from build123d import *

# Parameters (mm, degrees)
SKETCH_1_R          = 4.5
SKETCH_1_R_2        = 2.05
EXTRUDE_1_DEPTH     = 6
SKETCH_2_R          = 4
CUT_EXTRUDE_1_DEPTH = 2
SKETCH_3_R          = 6.65
CUT_EXTRUDE_2_DEPTH = 3.9
SKETCH_4_R          = 7.65
CUT_EXTRUDE_3_DEPTH = 1.5
SKETCH_5_R          = 6
SKETCH_5_R_2        = 2.05
EXTRUDE_2_DEPTH     = 5.1


with BuildPart() as part:
    # 草图1 → 凸台-拉伸1 (new body)
    with BuildSketch(Plane(origin=(0, 0, 0), x_dir=(1, 0, 0), z_dir=(0, 1, 0))):
        with BuildLine():
            Line((-14.168368772, -10.096516067), (29.831631228, -10.096516067))
            ThreePointArc((29.831631228, -10.096516067), (35.831631228, -4.096516067), (29.831631228, 1.903483933))
            Line((29.831631228, 1.903483933), (20.297540319, 1.903483933))
            ThreePointArc((20.297540319, 1.903483933), (16.762006413, 3.367950028), (15.297540319, 6.903483933))
            Line((15.297540319, 6.903483933), (15.297540319, 13.790407079))
            ThreePointArc((15.297540319, 13.790407079), (3.297540319, 25.790407079), (-8.702459681, 13.790407079))
            Line((-8.702459681, 13.790407079), (-8.702459681, 6.903483933))
            ThreePointArc((-8.702459681, 6.903483933), (-10.166925775, 3.367950028), (-13.702459681, 1.903483933))
            Line((-13.702459681, 1.903483933), (-14.168368772, 1.903483933))
            ThreePointArc((-14.168368772, 1.903483933), (-20.168368772, -4.096516067), (-14.168368772, -10.096516067))
        make_face()
        with Locations(Location((3.297540319, 13.790407079, 0), (0, 0, 270))):
            Circle(SKETCH_1_R, mode=Mode.SUBTRACT)
        with Locations(Location((-14.168368772, -4.096516067, 0), (0, 0, 270))):
            Circle(SKETCH_1_R_2, mode=Mode.SUBTRACT)
        with Locations(Location((29.831631228, -4.096516067, 0), (0, 0, 270))):
            Circle(SKETCH_1_R_2, mode=Mode.SUBTRACT)
    extrude(amount=EXTRUDE_1_DEPTH)

    # 草图2 → 切除-拉伸1 (cut)
    with BuildSketch(Plane.XZ):
        with Locations(Location((-14.168368772, 4.096516067, 0), (0, 0, 270))):
            Circle(SKETCH_2_R)
        with Locations(Location((29.831631228, 4.096516067, 0), (0, 0, 270))):
            Circle(SKETCH_2_R)
    extrude(amount=-CUT_EXTRUDE_1_DEPTH, mode=Mode.SUBTRACT)

    # 草图3 → 切除-拉伸2 (cut)
    with BuildSketch(Plane(origin=(0, 6, 0), x_dir=(1, 0, 0), z_dir=(0, 1, 0))):
        with Locations(Location((3.297540319, 13.790407079, 0), (0, 0, 270))):
            Circle(SKETCH_3_R)
    extrude(amount=-CUT_EXTRUDE_2_DEPTH, mode=Mode.SUBTRACT)

    # 草图4 → 切除-拉伸3 (cut)
    with BuildSketch(Plane(origin=(0, 6, 0), x_dir=(1, 0, 0), z_dir=(0, 1, 0))):
        with Locations(Location((3.297540319, 13.790407079, 0), (0, 0, 270))):
            Circle(SKETCH_4_R)
    extrude(amount=-CUT_EXTRUDE_3_DEPTH, mode=Mode.SUBTRACT)

    # 草图5 → 凸台-拉伸2 (add)
    with BuildSketch(Plane(origin=(0, 6, 0), x_dir=(1, 0, 0), z_dir=(0, 1, 0))):
        with Locations(Location((29.831631228, -4.096516067, 0), (0, 0, 270))):
            Circle(SKETCH_5_R)
        with Locations(Location((29.831631228, -4.096516067, 0), (0, 0, 90))):
            Circle(SKETCH_5_R_2, mode=Mode.SUBTRACT)
    extrude(amount=EXTRUDE_2_DEPTH)


solid = part.part
Read the model definition and answer for the solid it produces. Units are mm, in the model's axes. A direction names the side the tool comes from. Give positions to 0.01 mm unless a question says otherwise; leave off trailing zeros. Write each loop counter-clockwise with the first axis right and the second up, starting at its lowest first coordinate (ties: lowest second). Pieces come first, ordered by that corner, then holes. Notation, with made-up numbers: (-2, 27.25) - (26, 27.25) arc R21 ccw to (26, 38.25) - close; hole circle Ø10 at (41, 72). An arc over 180 degrees is marked (long way). Return JSON: item names as keys, results as strings.
Q1. A cutting plane is placed at D-D, the plane z = 4. Determine the outline of the cut face in (x, y), and give its area (3 significant figures).
Reply:
{"outline": "(-20.17, 0) - (-18.17, 0) - (-18.17, 2) - (-16.22, 2) - (-16.22, 6) - (-20.17, 6) - close; (-12.12, 2) - (-10.17, 2) - (-10.17, 0) - (25.83, 0) - (25.83, 2) - (27.78, 2) - (27.78, 11.1) - (23.83, 11.1) - (23.83, 6) - (-12.12, 6) - close; (31.88, 2) - (33.83, 2) - (33.83, 0) - (35.83, 0) - (35.83, 11.1) - (31.88, 11.1) - close", "area": "312 mm²"}
Q2. A cutting plane is placed at B-B, the plane z = -10.5. Determine the outline of the cut face in (x, y).
Reply:
{"outline": "(-8.7, 0) - (0.23, 0) - (0.23, 2.1) - (-2.48, 2.1) - (-2.48, 4.5) - (-3.61, 4.5) - (-3.61, 6) - (-8.7, 6) - close; (6.37, 0) - (15.3, 0) - (15.3, 6) - (10.2, 6) - (10.2, 4.5) - (9.08, 4.5) - (9.08, 2.1) - (6.37, 2.1) - close"}
Q3. A cutting plane is placed at C-C, the plane x = 30.5. Determine the outline of the cut face in (y, z).
Reply:
{"outline": "(0, -1.87) - (11.1, -1.87) - (11.1, 2.16) - (2, 2.16) - (2, 0.15) - (0, 0.15) - close; (0, 8.04) - (2, 8.04) - (2, 6.03) - (11.1, 6.03) - (11.1, 10.06) - (0, 10.06) - close"}
Q4. A cutting plane is placed at A-A, the plane y = 3. Determine the outline of the cut face in (x, z), and give its area (3 significant figures).
Reply:
{"outline": "(-14.17, -1.9) - (-13.7, -1.9) arc R5 cw to (-8.7, -6.9) - (-8.7, -13.79) arc R12 ccw to (15.3, -13.79) - (15.3, -6.9) arc R5 cw to (20.3, -1.9) - (29.83, -1.9) arc R6 ccw to (29.83, 10.1) - (-14.17, 10.1) arc R6 ccw to start; hole circle Ø4.1 at (-14.17, 4.1); hole circle Ø13.3 at (3.3, -13.79); hole circle Ø4.1 at (29.83, 4.1)", "area": "998 mm²"}
Q5. For a pull along Z with two mould halves and no side action, classify faces 6 (the face through (0.368, 5.26, -6.724)), 7 (the face through (-20.167, 2.958, 3.965)), 8 (the face through (-10.128, 2.958, -3.407)), 9 (the face through (0.56, 1.04, -17.36)) as released by +Z, released by -Z, zero draft, split by the parting line, or undercut.
Reply:
{"face 6": "undercut", "face 7": "split by the parting line", "face 8": "released by -Z", "face 9": "undercut"}
Q6. Given P1, Ø4, axis at x = 20.5, y = 2, coming from the -Z side; P2, Ø4, axis at x = 28.5, z = 4, coming from the -Y side; P3, Ø11, axis at x = -6.5, z = 0, coming from the +Y side, each flat-ended and moving along its own axis, determine where each tip first touches the part or whether it passes through.
Reply:
{"P1": "z = -2.24", "P2": "y = 2", "P3": "y = 6"}
Q7. For faces 1 (the face through (-16.17, 3.97, 3.65)), 2 (the face through (-17.717, 0.986, 2.251)), 3 (the face through (25, 3, -1.903)), 4 (the face through (-8.702, 3, -10)), 5 (the face through (10, 4.5, -16)), determine the directions among +Z, -Z, +X, -X, +Y, -Y from which every point of the face is accessible in a straight line to the end or side of a thin tool.
Reply:
{"face 1": "+Y, -Y", "face 2": "-Y", "face 3": "-Z, +X, +Y, -Y", "face 4": "-Z, -X, +Y, -Y", "face 5": "+Y"}
Q8. Consider line 1 along Z through (x, y) = (-14, 2.5); line 2 along X through (y, z) = (1.5, -8); line 3 along Y through (x, z) = (-14, -0.5). Determine where each line is inside the solid, lowest interval first. Write a range as [from, to].
Reply:
{"line 1": "[-1.9, 2.05], [6.14, 10.1]", "line 2": "[-8.7, 15.3]", "line 3": "[0, 6]"}
